Design review of the part built by this model. Coordinates are the model's own, in mm. A direction names the side the tool comes from. Round coordinates to 2 decimals unless told otherwise and drop trailing zeros. Loops run counter-clockwise (first coordinate to the right, second up) from the corner with the lowest first, then second, coordinate; pieces in that order, holes last. Notation, with made-up numbers: M 28,38 L 68,38 A7 ccw 68,51 Z; hole C -10.5,46.5 d5. An arc over 180 degrees is marked long. Use a Markdown table: item, result.
from build123d import *

# Parameters (mm, degrees)
F1_DEPTH = 170
F2_T     = -0.5


# Not quite as in the source:
# - a feature names something its author has since deleted; it is built from what else it names


with BuildPart() as f1:
    # F0 (on Top) → F1 (new body)
    with BuildSketch(Plane.XY):
        Polygon((16.3101451046, 28.25), (-16.3101451046, 28.25), (-32.6202902092, 0), (-16.3101451046, -28.25), (16.3101451046, -28.25), (32.6202902092, 0), align=None)
    extrude(amount=F1_DEPTH)

    # F2
    f2_openings = [f1.faces().sort_by_distance(p)[0] for p in [
        (0, 0, 170),
    ]]
    offset(amount=F2_T, openings=f2_openings)

    # F3: F1 across face


with BuildPart() as f1_1:
    add(f1.part)
    add(f1.part.mirror(Plane(origin=(-24.032204955, 13.875, 85.25), x_dir=(0.5, 0.8660254038, 0), z_dir=(0.8660254038, -0.5, 0))))


solid = f1_1.part
1. The part is to be moulded in two halves that separate along Y. For faces 1 (the face through (-72.21, 41.43, 84.06)), 2 (the face through (0, -28.25, 84)), 3 (the face through (1, 28.25, 84)), say which applies: pulls with the +Y half, pulls with the -Y half, needs draft (parallel to the pull), parting line crosses it, or undercut.
Check values:
| item | result |
|---|---|
| face 1 | undercut |
| face 2 | pulls with the -Y half |
| face 3 | pulls with the +Y half |
2. Take a section at D-D on y = 50.5. Give the boundary of the cut face in (x, z), and give its area (3 significant figures).
Check values:
| item | result |
|---|---|
| outline | M -67.55,0 L -28.58,0 L -28.58,170 L -29.16,170 L -29.16,0.5 L -66.97,0.5 L -66.97,170 L -67.55,170 Z |
| area | 215 mm² |
3. Take a section at B-B on x = -61.5. Give the boundary of the cut face in (y, z).
Check values:
| item | result |
|---|---|
| outline | M -0.5,0 L 56,0 L 56,170 L 55.5,170 L 55.5,0.5 L 0,0.5 L 0,170 L -0.5,170 Z |
4. Wall thickness on line 1 along Y through (x, z) = (11.5, 82.5); line 2 along Y through (x, z) = (-37, 101); line 3 along X through (y, z) = (27.5, 141.5): over which ranges is each line inside the solid? List them lowest first. Write a range as from..to.
Check values:
| item | result |
|---|---|
| line 1 | y = -28.25..-27.75, 27.75..28.25 |
| line 2 | y = -0.5..0, 55.5..56 |
| line 3 | x = -80.54..-79.96, -16.74..-15.59, 16.17..16.74 |
5. Insertion check: pin 1 (4 mm diameter, centred on x = -13, z = 133.5, fed in from +Y); pin 2 (6 mm diameter, centred on y = -12, z = 137, fed in from -X); pin 3 (1 mm diameter, centred on x = -1, y = 18.5, fed in from +Z); pin 4 (8 mm diameter, centred on x = -34.5, y = 0.5, fed in from -Z). Each pin has a flat end and moves straight along its axis. Give the tip position at first contact, or say it passes through.
Check values:
| item | result |
|---|---|
| pin 1 | stops at y = 28.25 |
| pin 2 | stops at x = -27.42 |
| pin 3 | stops at z = 0.5 |
| pin 4 | stops at z = 0 |
6. Machinability: for faces 4 (the face through (24.58, 13.93, 83.81)), 5 (the face through (-24, -13.93, 84.06)), 6 (the face through (-48, -0.5, 84)), which of the approach directions +Z, -Z, +X, -X, +Y, -Y give a long, thin tool a straight path to every point of the face, cutting with its end or side? Answer none if there is none.
Check values:
| item | result |
|---|---|
| face 4 | +Z, -Z, +X, +Y |
| face 5 | +Z |
| face 6 | +Z, -Z, -X, -Y |
7. Take a section at A-A on z = 65. Give the boundary of the cut face in (x, y), and give its area (3 significant figures).
Check values:
| item | result |
|---|---|
| outline | M -80.68,27.75 L -64.37,-0.5 L -32.33,-0.5 L -16.31,-28.25 L 16.31,-28.25 L 32.62,0 L 16.31,28.25 L -15.73,28.25 L -31.75,56 L -64.37,56 Z; hole M -80.11,27.75 L -64.09,0 L -32.62,0 L -16.31,28.25 L -32.04,55.5 L -64.09,55.5 Z; hole M -31.75,-0.5 L -16.02,-27.75 L 16.02,-27.75 L 32.04,0 L 16.02,27.75 L -15.44,27.75 Z |
| area | 193 mm² |
8. Take a section at C-C on y = 12. Give the boundary of the cut face in (x, z).
Check values:
| item | result |
|---|---|
| outline | M -71.59,0 L 25.69,0 L 25.69,170 L 25.11,170 L 25.11,0.5 L -24.54,0.5 L -24.54,170 L -25.69,170 L -25.69,0.5 L -71.01,0.5 L -71.01,170 L -71.59,170 Z |
